Autodesk Inventor part; units mm, degrees
ref_plane "YZ Plane" through (0, 0, 0) normal (1, 0, 0) x (0, 1, 0)
ref_plane "XZ Plane" through (0, 0, 0) normal (0, 1, 0) x (-1, 0, 0)
ref_plane "XY Plane" through (0, 0, 0) normal (0, 0, 1) x (1, 0, 0)
sketch "Body" plane through (0, 0, 0) normal (0, 0, 1) x (1, 0, 0)
  line L0 (0, 0) -> (60, 0) construction
  line L1 (-7, 2) -> (-2, 8.5)
  line L2 (-2, 8.5) -> (53, 14)
  line L3 (53, 14) -> (67, 6.5)
  line L4 (67, 6.5) -> (67, -7)
  line L5 (67, -7) -> (-7, -7)
  line L6 (-7, -7) -> (-7, 2)
  dimension "d1" = 60
  dimension "d2" = 7
  dimension "d4" = 7
  dimension "d5" = 7
  dimension "d6" = 14
  dimension "d8" = 13.5
  dimension "d9" = 9
  dimension "d13" = 8.5
  dimension "d14" = 5
  dimension "d15" = 14
extrude "BodyFeature" add sketch "Body" along normal blind 4
fillet "FilletsFeature" radius 2 4 edges at (-7, -7, 2) (67, -7, 2) (-7, 2, 2) (67, 6.5, 2)
sketch "MountHoles" plane through (0, 0, 4) normal (0, 0, 1) x (1, 0, 0)
  circle A0 centre (1.2887, 0.4289) radius 3.25
  circle A1 centre (25.2886, 0.4803) radius 3.25
  circle A2 centre (58.3386, 1.9174) radius 3.25
hole "MountHolesFeature" at (1.2887, 0.4289, 4) at (25.2886, 0.4803, 4) at (58.3386, 1.9174, 4) direction (0, 0, -1) diameter 6 end through all
properties part number "SpineNeckLinkConnector"
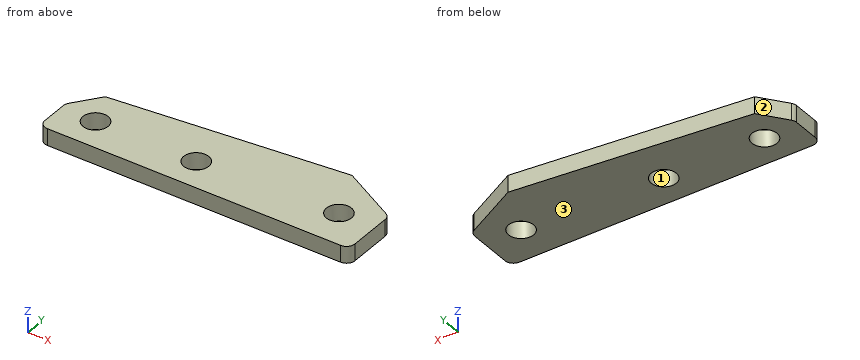
Geometry: final body of the model. Coordinates: model frame, mm. Face numbers are marked on the shaded views. Give positions to 0.01 mm unless a question says otherwise; leave off trailing zeros. Loops run counter-clockwise (first coordinate to the right, second up) from the corner with the lowest first, then second, coordinate; pieces in that order, holes last. Notation, with made-up numbers: (77.5, 29) -> (136.5, 29) arc R14 cw to (136.5, 36) -> close; hole circle Ø2 at (1.25, 9.5). An arc over 180 degrees is marked (long way). Put each result on its own line as item: value.
1. Cut plane A-A (y = 0). Return the cut outline in (x, z).
Taken from the geometry:
outline: (-7, 0) -> (-1.68, 0) -> (-1.68, 4) -> (-7, 4) -> close; (4.26, 0) -> (22.33, 0) -> (22.33, 4) -> (4.26, 4) -> close; (28.25, 0) -> (56.03, 0) -> (56.03, 4) -> (28.25, 4) -> close; (60.65, 0) -> (67, 0) -> (67, 4) -> (60.65, 4) -> close
2. Cut plane D-D (y = 12.5). Return the cut outline in (x, z), plus the area to 3 significant figures.
Taken from the geometry:
outline: (38, 0) -> (55.8, 0) -> (55.8, 4) -> (38, 4) -> close
area: 71.2 mm2
3. Pull-direction query (Y, two-part tool) for the marked faces 1, 2 and 3; classes: released by +Y, released by -Y, zero draft, split by the parting line, or undercut.
Taken from the geometry:
face 1: undercut
face 2: released by +Y
face 3: zero draft
4. Ray query, line 1 along X through (y, z) = (-2, 0.35); line 2 along X through (y, z) = (1.75, 1.8); line 3 along X through (y, z) = (2, 1.8). Return the intervals inside material, ascending. Write a range as [from, to].
Taken from the geometry:
line 1: x = [-7, -0.47], [3.05, 23.6], [26.98, 67]
line 2: x = [-6.95, -1.4], [3.98, 22.57], [28.01, 55.34], [61.33, 67]
line 3: x = [-6.88, -1.27], [3.84, 22.7], [27.88, 55.34], [61.34, 67]
5. Cut plane C-C (z = 2.4). Return the cut outline in (x, y).
Taken from the geometry:
outline: (-7, -5) arc R2 ccw to (-5, -7) -> (65, -7) arc R2 ccw to (67, -5) -> (67, 5.3) arc R2 ccw to (65.94, 7.07) -> (53, 14) -> (-2, 8.5) -> (-6.59, 2.54) arc R2 ccw to (-7, 1.32) -> close; hole circle Ø6 at (1.29, 0.43); hole circle Ø6 at (25.29, 0.48); hole circle Ø6 at (58.34, 1.92)
6. Cut plane B-B (x = 2.5). Return the cut outline in (y, z), plus the area to 3 significant figures.
Taken from the geometry:
outline: (-7, 0) -> (-2.32, 0) -> (-2.32, 4) -> (-7, 4) -> close; (3.17, 0) -> (8.95, 0) -> (8.95, 4) -> (3.17, 4) -> close
area: 41.8 mm2
